For this review, take the finished solid that the model builds, in its own axes (mm). Face numbers are marked on the shaded views. A direction names the side the tool comes from. Give positions to 0.01 mm unless a question says otherwise; leave off trailing zeros. Loops run counter-clockwise (first coordinate to the right, second up) from the corner with the lowest first, then second, coordinate; pieces in that order, holes last. Notation, with made-up numbers: M -15.5,65.25 L 39.5,65.25 A20 ccw 39.5,101.25 Z; hole C -35.75,80.5 d4. An arc over 180 degrees is marked long. Use CSV: the item, a comma, the result in double quotes. Start each with the question number.
1. Take a section at D-D, the plane x = 3. Write out the cut boundary in (y, z), and give its area (3 significant figures).
2. Tool access review of the marked faces 4 and 5: name each direction out of +Z, -Z, +X, -X, +Y, -Y from which nothing blocks a thin tool from reaching the whole face with its end or side.
3. Insertion check: P1, Ø4, axis at y = -7.5, z = -12.99, coming from the +X side; P2, Ø2, axis at x = 9, y = 10.5, coming from the -Z side; P3, Ø2, axis at x = 33.5, y = 11, coming from the +Z side. Each pin has a flat end and moves straight along its axis. Give the tip position at first contact, or say it passes through.
4. Take a section at B-B, the plane x = 40. Write out the cut boundary in (y, z).
5. Take a section at C-C, the plane z = 4. Write out the cut boundary in (x, y).
6. The part is to be moulded in two halves that separate along Z. For the marked faces 1, 2 and 3, say which applies: pulls with the +Z half, pulls with the -Z half, needs draft (parallel to the pull), parting line crosses it, or undercut.
7. Take a section at A-A, the plane y = 0. Write out the cut boundary in (x, z).
8. To check wall thickness, follow line 1 (Z direction, x = 35, y = -7.5); line 2 (Z direction, x = 34, y = -7) (3 decimals); line 3 (X direction, y = 13, z = 9.5). State the ranges of each line that lie inside material, in increasing order. Write a range as [from, to].
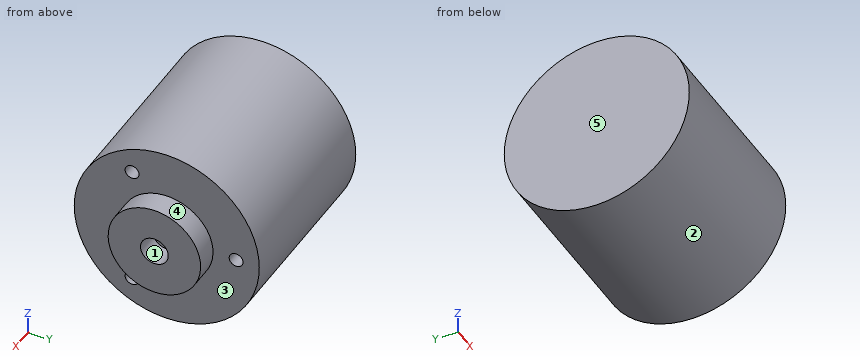
from build123d import *

# Parameters (mm, degrees)
SKETCH1_R                 = 20
BOSS_EXTRUDE1_DEPTH       = 39
SKETCH2_R                 = 10
BOSS_EXTRUDE2_DEPTH       = 5
F_3_0MM_DOWEL_HOLE1_D     = 3
F_3_0MM_DOWEL_HOLE1_DEPTH = 7
F_3_0MM_DOWEL_HOLE1_TIP   = 0.901290929
SKETCH3_R                 = 3
CUT_EXTRUDE2_DEPTH        = 5


with BuildPart() as part:
    # Sketch1 → Boss-Extrude1 (new body)
    with BuildSketch(Plane(origin=(0, 0, 0), x_dir=(0, 0, -1), z_dir=(1, 0, 0))):
        Circle(SKETCH1_R)
    extrude(amount=BOSS_EXTRUDE1_DEPTH)

    # Sketch2 → Boss-Extrude2 (add)
    with BuildSketch(Plane(origin=(39, 0, 0), x_dir=(0, 0, -1), z_dir=(1, 0, 0))):
        Circle(SKETCH2_R)
    extrude(amount=BOSS_EXTRUDE2_DEPTH)

    # Ø3.0mm Dowel Hole1
    with Locations(Plane(origin=(39, 15, 0), x_dir=(0, 0, 1), z_dir=(1, 0, 0))):
        with Locations((0, 0), (-12.990381057, 22.5), (12.990381057, 22.5)):
            Hole(F_3_0MM_DOWEL_HOLE1_D / 2, depth=F_3_0MM_DOWEL_HOLE1_DEPTH)
            with Locations((0, 0, -(F_3_0MM_DOWEL_HOLE1_DEPTH + F_3_0MM_DOWEL_HOLE1_TIP / 2))):  # 118° drill point
                Cone(0, F_3_0MM_DOWEL_HOLE1_D / 2, F_3_0MM_DOWEL_HOLE1_TIP, mode=Mode.SUBTRACT)

    # Sketch3 → Cut-Extrude2 (cut)
    with BuildSketch(Plane(origin=(44, 0, 0), x_dir=(0, 0, -1), z_dir=(1, 0, 0))):
        Circle(SKETCH3_R)
    extrude(amount=-CUT_EXTRUDE2_DEPTH, mode=Mode.SUBTRACT)


solid = part.part
Result set:
1,outline,"C 0,0 d40"
1,area,"1,260 mm2"
2,face 4,"+X"
2,face 5,"+Z, -Z, -X, +Y, -Y"
3,P1,"x = 39"
3,P2,"z = -17.6"
3,P3,"z = 17.32"
4,outline,"C 0,0 d20; hole C 0,0 d6"
5,outline,"M 0,-19.6 L 39,-19.6 L 39,-9.17 L 44,-9.17 L 44,9.17 L 39,9.17 L 39,19.6 L 0,19.6 Z"
6,face 1,"undercut"
6,face 2,"parting line crosses it"
6,face 3,"needs draft"
7,outline,"M 0,-20 L 39,-20 L 39,-10 L 44,-10 L 44,-3 L 39,-3 L 39,3 L 44,3 L 44,10 L 39,10 L 39,20 L 0,20 Z"
8,line 1,"[-18.54, -14.49], [-11.49, 11.49], [14.49, 18.54]"
8,line 2,"[-18.735, -14.405], [-11.576, 11.576], [14.405, 18.735]"
8,line 3,"[0, 39]"
